```python
from build123d import *

# Parameters (mm, degrees)
SKETCH1_R           = 5.15
SKETCH1_R_2         = 1.5
BOSS_EXTRUDE1_DEPTH = 11
SKETCH2_R           = 2.5
CUT_EXTRUDE1_DEPTH  = 6


with BuildPart() as part:
    # Sketch1 → Boss-Extrude1 (new body)
    with BuildSketch(Plane.XY):
        with BuildLine():
            Line((-21.4, -6.4), (-11.4, -6.4))
            Line((-11.4, -6.4), (-11.4, 0))
            ThreePointArc((-11.4, 0), (0, 11.4), (11.4, 0))
            Line((11.4, 0), (11.4, -6.4))
            Line((11.4, -6.4), (21.4, -6.4))
            Line((21.4, -6.4), (21.4, -11.4))
            Line((21.4, -11.4), (-21.4, -11.4))
            Line((-21.4, -11.4), (-21.4, -6.4))
        make_face()
        Circle(SKETCH1_R, mode=Mode.SUBTRACT)
        with Locations((-5.656854249, 5.656854249)):
            Circle(SKETCH1_R_2, mode=Mode.SUBTRACT)
        with Locations((5.656854249, 5.656854249)):
            Circle(SKETCH1_R_2, mode=Mode.SUBTRACT)
        with Locations((-5.656854249, -5.656854249)):
            Circle(SKETCH1_R_2, mode=Mode.SUBTRACT)
        with Locations((5.656854249, -5.656854249)):
            Circle(SKETCH1_R_2, mode=Mode.SUBTRACT)
    extrude(amount=BOSS_EXTRUDE1_DEPTH)

    # Sketch2 → Cut-Extrude1 (cut, through all)
    with BuildSketch(Plane(origin=(0, -6.4, 0), x_dir=(1, 0, 0), z_dir=(0, 1, 0))):
        with Locations((-15.9, -5.5)):
            Circle(SKETCH2_R)
        with Locations((15.9, -5.5)):
            Circle(SKETCH2_R)
    extrude(amount=-CUT_EXTRUDE1_DEPTH, mode=Mode.SUBTRACT)


solid = part.part
```
Work out the finished part from the listing and answer in its coordinate system (mm). A direction names the side the tool comes from. Round coordinates to 2 decimals unless told otherwise and drop trailing zeros. Write each loop counter-clockwise with the first axis right and the second up, starting at its lowest first coordinate (ties: lowest second). Pieces come first, ordered by that corner, then holes.
1) A cutting plane is placed at D-D on y = -8.75. Determine the outline of the cut face in (x, z), and give its area (3 significant figures).
2) Consider probe 1 along Y at (x, z) = (0, 4.75); probe 2 along X at (y, z) = (-9.25, 4.5); probe 3 along X at (y, z) = (0.25, 1.75). Determine where each line is inside the solid, lowest interval first.
3) Which of the six approach directions +Z, -Z, +X, -X, +Y, -Y give full straight-line access (tool end or side, diameter ignored) to faces 1 (the face through (-11.4, -3, 5)), 2 (the face through (19, -6.4, 5)), 3 (the face through (-0.251, 11.397, 5.423))?
4) Determine the mould class of faces 4 (the face through (0, -7, 11)), 5 (the face through (18.285, -8.865, 4.749)), 6 (the face through (6.3, 4.3, 5.4)), 7 (the face through (-16, -9, 3)) for opening direction Z: pulls with the +Z half, pulls with the -Z half, needs draft (parallel to the pull), parting line crosses it, or undercut.
5) A cutting plane is placed at C-C on x = 1. Determine the outline of the cut face in (y, z).
6) Flat-ended cylindrical pins translate along their axes: P1, Ø2, axis at y = 7, z = 1.5, coming from the +X side; P2, Ø4, axis at x = 7, z = 5.5, coming from the +Y side (3 decimals); P3, Ø12, axis at x = 0, y = 0, coming from the +Z side; P4, Ø2.5, axis at x = 5.66, y = -5.66, coming from the +Z side. Find the tip coordinate at first contact, or state that the pin passes through.
7) A cutting plane is placed at B-B on y = -2.25. Determine the outline of the cut face in (x, z), and give its area (3 significant figures).
8) A cutting plane is placed at A-A on x = 6. Determine the outline of the cut face in (y, z), and give its area (3 significant figures).
Entries:
1. outline: (-21.4, 0) - (21.4, 0) - (21.4, 11) - (-21.4, 11) - close; hole circle Ø5 at (-15.9, 5.5); hole circle Ø5 at (15.9, 5.5)
1. area: 432 mm2
2. probe 1: y = -11.4 to -5.15, 5.15 to 11.4
2. probe 2: x = -21.4 to -18.19, -13.61 to 13.61, 18.19 to 21.4
2. probe 3: x = -11.4 to -5.14, 5.14 to 11.4
3. face 1: +Z, -Z, -X, +Y
3. face 2: +Z, -Z, +X, +Y
3. face 3: +Z, -Z, +Y
4. face 4: pulls with the +Z half
4. face 5: undercut
4. face 6: needs draft
4. face 7: undercut
5. outline: (-11.4, 0) - (-5.05, 0) - (-5.05, 11) - (-11.4, 11) - close; (5.05, 0) - (11.36, 0) - (11.36, 11) - (5.05, 11) - close
6. P1: stops at x = 9.69
6. P2: stops at y = 10.245
6. P3: stops at z = 11
6. P4: passes through
7. outline: (-11.4, 0) - (-4.63, 0) - (-4.63, 11) - (-11.4, 11) - close; (4.63, 0) - (11.4, 0) - (11.4, 11) - (4.63, 11) - close
7. area: 149 mm2
8. outline: (-11.4, 0) - (-7.12, 0) - (-7.12, 11) - (-11.4, 11) - close; (-4.2, 0) - (4.2, 0) - (4.2, 11) - (-4.2, 11) - close; (7.12, 0) - (9.69, 0) - (9.69, 11) - (7.12, 11) - close
8. area: 168 mm2
